Here's how the part is built. I have some questions about the finished solid (model axes, mm). Face numbers are marked on the shaded views. Coordinates: 2 decimals unless noted, no trailing zeros. Write each loop counter-clockwise with the first axis right and the second up, starting at its lowest first coordinate (ties: lowest second). Pieces come first, ordered by that corner, then holes.
(1) Please list where these lines run through material, in increasing order: probe 1 along Z at (x, y) = (-2.5, -94); probe 2 along Z at (x, y) = (-5, -22.5); probe 3 along Y at (x, z) = (-9, -7).
(2) Imagine slicing it at A-A, the plane x = -3. List the corners of the cut face in (y, z) for me, plus the area to 3 significant figures.
(3) Imagine slicing it at B-B, the plane y = -57. State how many separate pieces and enclosed holes the cut face has, plus the area to 3 significant figures.
(4) For pin 1 Ø2 at (x, z) = (-6.5, -142.5) entering from -Y; pin 2 Ø24 at (y, z) = (-14, -19) entering from -X, each with a flat end and sliding along its axis, tell me the tip position at first contact or that it passes through.
(5) Imagine slicing it at D-D, the plane z = -138. List the corners of the cut face in (x, y) for me.
(6) Thinking about a two-plate mould opening in Z: for the marked faces 1 and 2, which applies, released by +Z, released by -Z, zero draft, split by the parting line, or undercut?
(7) Imagine slicing it at C-C, the plane y = -9. List the corners of the cut face in (x, z) for me, plus the area to 3 significant figures.
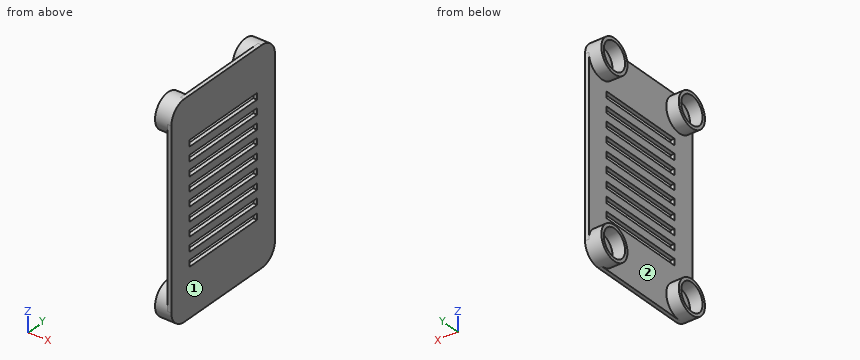
Autodesk Fusion 360 part; units mm, degrees
sketch "Esquisse1" plane through (0, 0, 0) normal (1, 0, 0) x (0, 0, -1)
  line L0 (-0.0946, -0.1527) -> (166.9054, -0.1527)
  line L1 (166.9054, -0.1527) -> (166.9054, -107.1527)
  line L2 (166.9054, -107.1527) -> (-0.0946, -107.1527)
  line L3 (-0.0946, -107.1527) -> (-0.0946, -0.1527)
  circle A0 centre (153.4054, -13.6527) radius 11
  circle A1 centre (13.4054, -13.6527) radius 11
  circle A2 centre (13.4054, -93.6527) radius 11
  circle A3 centre (153.4054, -93.6527) radius 11
  circle A4 centre (153.4054, -13.6527) radius 13.5
  circle A5 centre (153.4054, -93.6527) radius 13.5
  circle A6 centre (13.4054, -93.6527) radius 13.5
  circle A7 centre (13.4054, -13.6527) radius 13.5
  dimension "d10" = 107
  dimension "d11" = 167
  dimension "d12" = 22
  dimension "d13" = 13.5
  dimension "d14" = 13.5
  dimension "d15" = 22
  dimension "d16" = 22
  dimension "d17" = 22
  dimension "d18" = 13.5
  dimension "d19" = 13.5
  dimension "d20" = 13.5
  dimension "d21" = 13.5
  dimension "d22" = 13.5
  dimension "d23" = 13.5
  dimension "d24" = 27
  dimension "d25" = 27
  dimension "d26" = 27
  dimension "d27" = 27
extrude "Extrusion1" add sketch "Esquisse1" along normal blind 3 contours L0 L1 L2 L3 A4 A5 A6 A7 | A7 | A4 | A6 | A5 | A0 | A1 | A2 | A3
extrude "Extrusion2" add sketch "Esquisse1" against normal blind 10 contours A7 | A4 | A6 | A5
sketch "Esquisse3" plane through (0, 0, 0) normal (-1, 0, 0) x (0, 0, 1)
  arc A0 (-166.9054, -13.6527) -> (-153.4054, -0.1527) centre (-153.4054, -13.6527) ccw
  line L0 (-166.9054, -13.6527) -> (-166.9054, -93.6527)
  arc A1 (-153.4054, -107.1527) -> (-166.9054, -93.6527) centre (-153.4054, -93.6527) ccw
  line L1 (-153.4054, -107.1527) -> (-13.4054, -107.1527)
  arc A2 (0.0946, -93.6527) -> (-13.4054, -107.1527) centre (-13.4054, -93.6527) ccw
  line L2 (0.0946, -93.6527) -> (0.0946, -13.6527)
  arc A3 (-13.4054, -0.1527) -> (0.0946, -13.6527) centre (-13.4054, -13.6527) ccw
  line L3 (-13.4054, -0.1527) -> (-153.4054, -0.1527)
  line L4 (-78.4054, -88.6527) -> (-83.4054, -88.6527)
  line L5 (-83.4054, -88.6527) -> (-83.4054, -18.6527)
  line L6 (-83.4054, -18.6527) -> (-78.4054, -18.6527)
  line L7 (-78.4054, -18.6527) -> (-78.4054, -88.6527)
  line L8 (-72.1554, -88.6527) -> (-72.1554, -18.6527)
  line L9 (-67.1554, -88.6527) -> (-72.1554, -88.6527)
  line L10 (-67.1554, -18.6527) -> (-67.1554, -88.6527)
  line L11 (-72.1554, -18.6527) -> (-67.1554, -18.6527)
  line L12 (-60.9054, -88.6527) -> (-60.9054, -18.6527)
  line L13 (-55.9054, -88.6527) -> (-60.9054, -88.6527)
  line L14 (-55.9054, -18.6527) -> (-55.9054, -88.6527)
  line L15 (-60.9054, -18.6527) -> (-55.9054, -18.6527)
  line L16 (-49.6554, -88.6527) -> (-49.6554, -18.6527)
  line L17 (-44.6554, -88.6527) -> (-49.6554, -88.6527)
  line L18 (-44.6554, -18.6527) -> (-44.6554, -88.6527)
  line L19 (-49.6554, -18.6527) -> (-44.6554, -18.6527)
  line L20 (-38.4054, -88.6527) -> (-38.4054, -18.6527)
  line L21 (-33.4054, -88.6527) -> (-38.4054, -88.6527)
  line L22 (-33.4054, -18.6527) -> (-33.4054, -88.6527)
  line L23 (-38.4054, -18.6527) -> (-33.4054, -18.6527)
  line L24 (-94.6554, -88.6527) -> (-94.6554, -18.6527)
  line L25 (-89.6554, -18.6527) -> (-89.6554, -88.6527)
  line L26 (-89.6554, -88.6527) -> (-94.6554, -88.6527)
  line L27 (-94.6554, -18.6527) -> (-89.6554, -18.6527)
  line L28 (-105.9054, -88.6527) -> (-105.9054, -18.6527)
  line L29 (-100.9054, -18.6527) -> (-100.9054, -88.6527)
  line L30 (-100.9054, -88.6527) -> (-105.9054, -88.6527)
  line L31 (-105.9054, -18.6527) -> (-100.9054, -18.6527)
  line L32 (-117.1554, -88.6527) -> (-117.1554, -18.6527)
  line L33 (-112.1554, -18.6527) -> (-112.1554, -88.6527)
  line L34 (-112.1554, -88.6527) -> (-117.1554, -88.6527)
  line L35 (-117.1554, -18.6527) -> (-112.1554, -18.6527)
  line L36 (-128.4054, -88.6527) -> (-128.4054, -18.6527)
  line L37 (-123.4054, -18.6527) -> (-123.4054, -88.6527)
  line L38 (-123.4054, -88.6527) -> (-128.4054, -88.6527)
  line L39 (-128.4054, -18.6527) -> (-123.4054, -18.6527)
  dimension "d35" = 5
  dimension "d36" = 70
  dimension "d37" = 83.5
  dimension "d38" = 18.5
  dimension "d41" = 45
  dimension "d42" = 0
  dimension "d45" = -45
  dimension "d46" = 0
extrude "Extrusion3" cut sketch "Esquisse3" against normal blind 25 contours L4 L5 L6 L7 | L8 L9 L10 L11 | L12 L13 L14 L15 | L16 L17 L18 L19 | L20 L21 L22 L23 | L24 L25 L26 L27 | L28 L29 L30 L31 | L32 L33 L34 L35 | L36 L37 L38 L39
equation "diaPiedBois = 22 mm"
equation "longEntrePied = 140 mm"
equation "largEntrePied = 80 mm"
equation "d10 = largEntrePied + diaExtPiedBois"
equation "d11 = longEntrePied + diaExtPiedBois"
equation "d12 = diaPiedBois"
equation "d13 = diaExtPiedBois / 2"
equation "d14 = diaExtPiedBois / 2"
equation "d15 = diaPiedBois"
equation "d16 = diaPiedBois"
equation "d17 = diaPiedBois"
equation "d18 = diaExtPiedBois / 2"
equation "d19 = diaExtPiedBois / 2"
equation "d20 = diaExtPiedBois / 2"
equation "d21 = diaExtPiedBois / 2"
equation "d22 = diaExtPiedBois / 2"
equation "d23 = diaExtPiedBois / 2"
equation "d24 = diaPiedBois + 5 mm"
equation "d25 = diaPiedBois + 5 mm"
equation "d26 = diaPiedBois + 5 mm"
equation "d27 = diaPiedBois + 5 mm"
equation "diaExtPiedBois = diaPiedBois + 5 mm"
equation "d29 = epPlaqueHaut"
equation "epPlaqueHaut = 3 mm"
equation "hautSupportPiedBois = 10 mm"
equation "d37 = ( longEntrePied + diaExtPiedBois ) / 2"
equation "d38 = ( largEntrePied + diaExtPiedBois ) / 2 - ( 70 / 2 ) * 1 mm"
Recorded:
1. probe 1: z = -166.9 to -164.4, -142.41 to -139.91, -26.9 to -24.4, -2.41 to 0.09
1. probe 2: z = -163.6 to -159.94, -146.87 to -143.21, -23.6 to -19.94, -6.87 to -3.21
1. probe 3: y = -105.54 to -102.6, -84.71 to -81.77, -25.54 to -22.6, -4.71 to -1.77
2. outline: circle Ø27 at (-93.65, -153.41); circle Ø27 at (-93.65, -13.41); circle Ø27 at (-13.65, -153.41); circle Ø27 at (-13.65, -13.41); hole circle Ø22 at (-93.65, -153.41); hole circle Ø22 at (-93.65, -13.41); hole circle Ø22 at (-13.65, -153.41); hole circle Ø22 at (-13.65, -13.41)
2. area: 770 mm2
3. separate pieces: 10
3. enclosed holes: 0
3. area: 366 mm2
4. pin 1: stops at y = -102.83
4. pin 2: stops at x = -10
5. outline: (0, -107.15) - (3, -107.15) - (3, -0.15) - (0, -0.15) - close
6. face 1: zero draft
6. face 2: undercut
7. outline: (-10, -166.08) - (3, -166.08) - (3, -0.73) - (-10, -0.73) - (-10, -3.44) - (0, -3.44) - (0, -23.37) - (-10, -23.37) - (-10, -26.08) - (0, -26.08) - (0, -140.73) - (-10, -140.73) - (-10, -143.44) - (0, -143.44) - (0, -163.37) - (-10, -163.37) - close
7. area: 604 mm2
